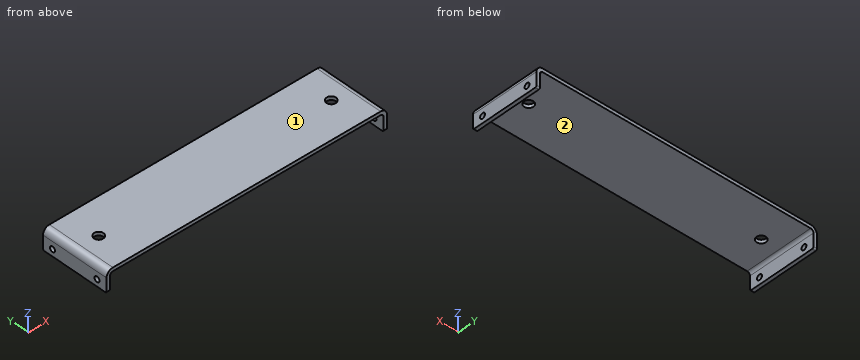
```python
from build123d import *

# Parameters (mm, degrees)
SKETCH1_W                        = 260.35
SKETCH1_H                        = 63.5
BASE_FLANGE1_DEPTH               = 3.2639
EDGE_FLANGE1_STRIP_W             = 18.36928
EDGE_FLANGE1_STRIP_H             = 3.2639
EDGE_FLANGE1_STRIP_CUT_DEPTH     = 63.5
EDGE_FLANGE1_STRIP_2_W           = 18.36928
EDGE_FLANGE1_STRIP_2_H           = 3.2639
EDGE_FLANGE1_STRIP_CUT_2_DEPTH   = 63.5
EDGE_FLANGE1_DEPTH               = 63.5
EDGE_FLANGE1_BEND_DEPTH          = 63.5
F_10_0_1935_DIAMETER_HOLE1_D     = 4.9149
FILLET1_R                        = 1.27
F_11_32_0_34375_DIAMETER_HOLE1_D = 8.73125


# Sheet-metal steps are written as plain solids
with BuildPart() as part:
    # Sketch1 → Base-Flange1 (new body)
    with BuildSketch(Plane.XY):
        Rectangle(SKETCH1_W, SKETCH1_H)
    extrude(amount=-BASE_FLANGE1_DEPTH)

    # Edge-Flange1 strip (across the edge) → Edge-Flange1 strip cut (cut)
    with BuildSketch(Plane(origin=(130.175, 31.75, -3.2639), x_dir=(-1, 0, 0), z_dir=(0, -1, 0))):
        with Locations((-3.2639, -1.63195)):
            Rectangle(EDGE_FLANGE1_STRIP_W, EDGE_FLANGE1_STRIP_H)
    extrude(amount=EDGE_FLANGE1_STRIP_CUT_DEPTH, mode=Mode.SUBTRACT)

    # Edge-Flange1 strip 2 (across the edge) → Edge-Flange1 strip cut 2 (cut)
    with BuildSketch(Plane(origin=(-130.175, -31.75, -3.2639), x_dir=(1, 0, 0), z_dir=(0, 1, 0))):
        with Locations((-3.2639, -1.63195)):
            Rectangle(EDGE_FLANGE1_STRIP_2_W, EDGE_FLANGE1_STRIP_2_H)
    extrude(amount=EDGE_FLANGE1_STRIP_CUT_2_DEPTH, mode=Mode.SUBTRACT)

    # Edge-Flange1 section (across the edge) → Edge-Flange1 (add)
    with BuildSketch(Plane(origin=(130.175, 31.75, -3.2639), x_dir=(-1, 0, 0), z_dir=(0, -1, 0))):
        with BuildLine():
            Line((0, 2.65684), (0, 15.7861))
            Line((0, 15.7861), (3.2639, 15.7861))
            Line((3.2639, 15.7861), (3.2639, 2.65684))
            ThreePointArc((3.2639, 2.65684), (4.042070419, 0.778170419), (5.92074, 0))
            Line((5.92074, 0), (5.92074, -3.2639))
            ThreePointArc((5.92074, -3.2639), (1.734144596, -1.529755404), (0, 2.65684))
        make_face()
    extrude(amount=EDGE_FLANGE1_DEPTH)

    # Edge-Flange1 section 2 (across the edge) → Edge-Flange1 bend (add)
    with BuildSketch(Plane(origin=(-130.175, -31.75, -3.2639), x_dir=(1, 0, 0), z_dir=(0, 1, 0))):
        with BuildLine():
            Line((0, 2.65684), (0, 15.7861))
            Line((0, 15.7861), (3.2639, 15.7861))
            Line((3.2639, 15.7861), (3.2639, 2.65684))
            ThreePointArc((3.2639, 2.65684), (4.042070419, 0.778170419), (5.92074, 0))
            Line((5.92074, 0), (5.92074, -3.2639))
            ThreePointArc((5.92074, -3.2639), (1.734144596, -1.529755404), (0, 2.65684))
        make_face()
    extrude(amount=EDGE_FLANGE1_BEND_DEPTH)

    # #10 (0.1935) Diameter Hole1 (through all)
    with Locations(Plane(origin=(130.175, 0, 0), x_dir=(0, 0, -1), z_dir=(1, 0, 0))):
        with Locations((12.7, 22.225), (12.7, -22.225)):
            Hole(F_10_0_1935_DIAMETER_HOLE1_D / 2)

    # Fillet1
    fillet1_edges = [part.edges().sort_by_distance(p)[0] for p in [
        (128.54305, 31.75, -19.05),
        (128.54305, -31.75, -19.05),
        (-128.54305, -31.75, -19.05),
        (-128.54305, 31.75, -19.05),
    ]]
    fillet(fillet1_edges, radius=FILLET1_R)

    # 11/32 (0.34375) Diameter Hole1 (through all)
    with Locations(Plane.XY):
        with Locations((-107.95, 0), (107.95, 0)):
            Hole(F_11_32_0_34375_DIAMETER_HOLE1_D / 2)


solid = part.part
```
Geometry: final body of the model. Coordinates: model frame, mm. Face numbers are marked on the shaded views. Give positions to 0.01 mm unless a question says otherwise; leave off trailing zeros. Write each loop counter-clockwise with the first axis right and the second up, starting at its lowest first coordinate (ties: lowest second). Pieces come first, ordered by that corner, then holes.
1. Draft query along X for the marked faces 1 and 2. Return one class per face: released by +X, released by -X, zero draft, split by the parting line, or undercut.
2. Section query D-D, the plane y = 17. Return loops of the section in (x, z) (3 decimals).
3. Line query: probe 1 along X at (y, z) = (-0.5, -12) (3 decimals); probe 2 along Y at (x, z) = (-128.6, -12.7); probe 3 along Y at (x, z) = (-108, -0.75). Output: solid intervals per line, ascending.
4. Section query C-C, the plane x = -107.95. Return loops of the section in (y, z), then the cut area to 3 significant figures.
5. Section query B-B, the plane y = 0. Return loops of the section in (x, z) (3 decimals), then the cut area to 3 significant figures.
6. Section query A-A, the plane z = -12.7. Return loops of the section in (x, y) (3 decimals).
7. Pin query (flat end, axial travel): P1, Ø1.5, axis at x = -25, y = -15.5, coming from the -Z side; P2, Ø1.5, axis at y = 4, z = -3.5, coming from the -X side; P3, Ø8, axis at x = 107.95, y = 0, coming from the -Z side. Return the tip coordinate at first contact, or that it passes through.
Computed:
1. face 1: zero draft
1. face 2: undercut
2. outline: (-130.175, -19.05) - (-126.911, -19.05) - (-126.911, -5.921) arc R2.657 cw to (-124.254, -3.264) - (124.254, -3.264) arc R2.657 cw to (126.911, -5.921) - (126.911, -19.05) - (130.175, -19.05) - (130.175, -5.921) arc R5.921 ccw to (124.254, 0) - (-124.254, 0) arc R5.921 ccw to (-130.175, -5.921) - close
3. probe 1: x = -130.175 to -126.911, 126.911 to 130.175
3. probe 2: y = -31.75 to -24.68, -19.77 to 19.77, 24.68 to 31.75
3. probe 3: y = -31.75 to -4.37, 4.37 to 31.75
4. outline: (-31.75, -3.26) - (-4.37, -3.26) - (-4.37, 0) - (-31.75, 0) - close; (4.37, -3.26) - (31.75, -3.26) - (31.75, 0) - (4.37, 0) - close
4. area: 179 mm2
5. outline: (-130.175, -19.05) - (-126.911, -19.05) - (-126.911, -5.921) arc R2.657 cw to (-124.254, -3.264) - (-112.316, -3.264) - (-112.316, 0) - (-124.254, 0) arc R5.921 ccw to (-130.175, -5.921) - close; (-103.584, -3.264) - (103.584, -3.264) - (103.584, 0) - (-103.584, 0) - close; (112.316, -3.264) - (124.254, -3.264) arc R2.657 cw to (126.911, -5.921) - (126.911, -19.05) - (130.175, -19.05) - (130.175, -5.921) arc R5.921 ccw to (124.254, 0) - (112.316, 0) - close
5. area: 884 mm2
6. outline: (-130.175, -31.75) - (-126.911, -31.75) - (-126.911, -24.682) - (-130.175, -24.682) - close; (-130.175, -19.768) - (-126.911, -19.768) - (-126.911, 19.768) - (-130.175, 19.768) - close; (-130.175, 24.682) - (-126.911, 24.682) - (-126.911, 31.75) - (-130.175, 31.75) - close; (126.911, -31.75) - (130.175, -31.75) - (130.175, -24.682) - (126.911, -24.682) - close; (126.911, -19.768) - (130.175, -19.768) - (130.175, 19.768) - (126.911, 19.768) - close; (126.911, 24.682) - (130.175, 24.682) - (130.175, 31.75) - (126.911, 31.75) - close
7. P1: stops at z = -3.26
7. P2: stops at x = -129.93
7. P3: passes through
